Build history of the part. All positions in model axes, mm. A direction names the side the tool comes from. Coordinates: 2 decimals unless noted, no trailing zeros. Order: outer loops, then holes, each group sorted by start corner. A loop starts at its lowest first (then second) coordinate and runs counter-clockwise, first axis right, second up. Notation, with made-up numbers: M -11,32.25 L 46,32.25 A13 ccw 46,55.25 Z; hole C 47,77.5 d11. An arc over 180 degrees is marked long. Use a Markdown table: item, result. Add a question column.
from build123d import *

# Parameters (mm, degrees)
BOSS_EXTRUDE1_DEPTH      = 90
BOSS_EXTRUDE1_DEPTH_BACK = 90
SKETCH1_W                = 252
SKETCH1_H                = 5
CUT_EXTRUDE1_DEPTH       = 220.732223399
SKETCH5_W                = 202
SKETCH5_H                = 130
CUT_EXTRUDE3_DEPTH       = 155.922561301


with BuildPart() as part:
    # Sketch1 → Boss-Extrude1 (new, two sides: drawn at the far end of the back side and taken through both)
    with BuildSketch(Plane.XY.offset(-BOSS_EXTRUDE1_DEPTH_BACK)):
        Rectangle(SKETCH1_W, SKETCH1_H)
    extrude(amount=BOSS_EXTRUDE1_DEPTH + BOSS_EXTRUDE1_DEPTH_BACK)

    # Sketch2 → Cut-Extrude1 (cut, through all)
    with BuildSketch(Plane.XY.offset(90)):
        Polygon((-21, 1.443375673), (-22.25, 0.721687836), (-22.25, -0.721687836), (-21, -1.443375673), (-19.75, -0.721687836), (-19.75, 0.721687836), align=None)
        Polygon((121, 1.443375673), (119.75, 0.721687836), (119.75, -0.721687836), (121, -1.443375673), (122.25, -0.721687836), (122.25, 0.721687836), align=None)
    extrude(amount=-CUT_EXTRUDE1_DEPTH, mode=Mode.SUBTRACT)

    # Sketch5 → Cut-Extrude3 (cut, through all)
    with BuildSketch(Plane(origin=(0, 2.5, 0), x_dir=(1, 0, 0), z_dir=(0, 1, 0))):
        Rectangle(SKETCH5_W, SKETCH5_H)
    extrude(amount=-CUT_EXTRUDE3_DEPTH, mode=Mode.SUBTRACT)


solid = part.part
(1) Mould opens along Z. For faces 3 (the flat face through (-1, 0, -65)), 4 (the flat face through (-2, 0, 90)), 5 (the flat face through (-2, 2.5, 79)), 6 (the flat face through (101, 0, 1)) say: released by +Z, released by -Z, zero draft, split by the parting line, or undercut.
(2) Drill centre lines: line 1 along X through (y, z) = (0.4, -26); line 2 along Z through (x, y) = (34, 0.3); line 3 along X through (y, z) = (0, -81). Where is each one in solid material? Low to high. Write a range as from..to.
(3) Slice it at B-B on x = -34. Give the cut face in (y, z).
(4) Slice it at A-A on z = -25.5. Give the cut face in (x, y).
(5) Which spindle directions (+Z, -Z, +X, -X, +Y, -Y) get a long thin tool onto all of the face, cutting with end or side? Do faces 1 (the flat face through (-1, 0, 65)), 2 (the flat face through (-2, -2.5, 79)). Say none if no direction does.
Solutions:
| question | item | result |
|---|---|---|
| 1 | face 3 | undercut |
| 1 | face 4 | released by +Z |
| 1 | face 5 | zero draft |
| 1 | face 6 | undercut |
| 2 | line 1 | -126..-101, 101..119.75, 122.25..126 |
| 2 | line 2 | -90..-65, 65..90 |
| 2 | line 3 | -126..-22.25, -19.75..119.75, 122.25..126 |
| 3 | outline | M -2.5,-90 L 2.5,-90 L 2.5,-65 L -2.5,-65 Z; M -2.5,65 L 2.5,65 L 2.5,90 L -2.5,90 Z |
| 4 | outline | M -126,-2.5 L -101,-2.5 L -101,2.5 L -126,2.5 Z; M 101,-2.5 L 126,-2.5 L 126,2.5 L 101,2.5 Z; hole M 119.75,-0.72 L 121,-1.44 L 122.25,-0.72 L 122.25,0.72 L 121,1.44 L 119.75,0.72 Z |
| 5 | face 1 | +Y, -Y |
| 5 | face 2 | +Z, -Z, +X, -X, -Y |
